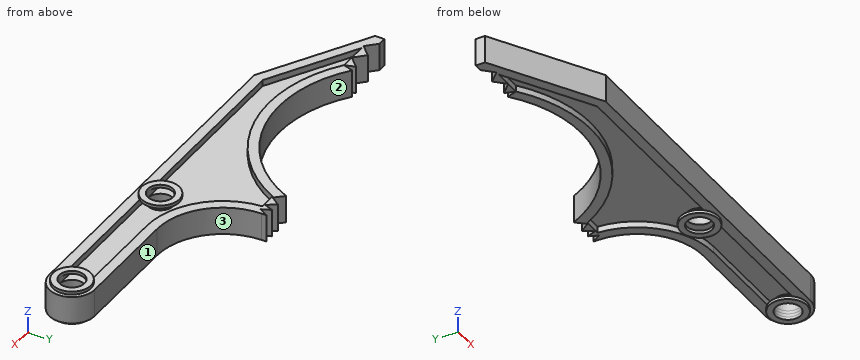
```python
from build123d import *

# Parameters (mm, degrees)
BOSS_EXTRUDE1_DEPTH     = 4
SKETCH3_R               = 2.5
CUT_EXTRUDE1_DEPTH      = 82.558227053
CUT_EXTRUDE2_DEPTH      = 1.25
SKETCH5_R               = 3.75
SKETCH5_R_2             = 2.5
BOSS_EXTRUDE2_DEPTH     = 0.625
CUT_EXTRUDE3_START      = -8
CUT_EXTRUDE3_DEPTH      = 8
CUT_EXTRUDE4_START      = -1.25
CUT_EXTRUDE4_DEPTH      = 1.25
CUT_EXTRUDE5_DEPTH      = 79.859241849
CUT_EXTRUDE5_DEPTH_BACK = 79.859241849
CUT_EXTRUDE6_DEPTH      = 79.859241849
CUT_EXTRUDE6_DEPTH_BACK = 79.859241849


# Read off the part's stored shape, not the designer's step: Cut-Extrude3
with BuildPart() as part:
    # Sketch1 → Boss-Extrude1 (new, symmetric)
    with BuildSketch(Plane.XY):
        with BuildLine():
            Line((0, 0), (70, 0))
            ThreePointArc((70, 0), (76.5, 6.5), (70, 13))
            Line((70, 13), (48.916352203, 13))
            ThreePointArc((48.916352203, 13), (41.053324797, 16.256972593), (37.796352203, 24.12))
            Line((37.796352203, 24.12), (37.796352203, 27.12))
            Line((37.796352203, 27.12), (27.786352203, 27.12))
            ThreePointArc((27.786352203, 27.12), (12.065558159, 13.089935965), (-8.483647797, 17.75))
            Line((-8.483647797, 17.75), (-22.083647797, 17.75))
            Line((-22.083647797, 17.75), (-22.083647797, 12.75))
            Line((-22.083647797, 12.75), (0, 0))
        make_face()
    extrude(amount=BOSS_EXTRUDE1_DEPTH, both=True)

    # Sketch3 → Cut-Extrude1 (cut, through all)
    with BuildSketch(Plane(origin=(0, 0, -4), x_dir=(-1, 0, 0), z_dir=(0, 0, -1))):
        with Locations((-70, 6.5)):
            Circle(SKETCH3_R)
        with Locations((-40, 6.5)):
            Circle(SKETCH3_R)
    extrude(amount=-CUT_EXTRUDE1_DEPTH, mode=Mode.SUBTRACT)

    # Sketch4 → Cut-Extrude2 (cut)
    with BuildSketch(Plane.XY.offset(4)):
        with BuildLine():
            Line((-20.083647797, 13.904700538), (0.535898385, 2))
            Line((0.535898385, 2), (70, 2))
            ThreePointArc((70, 2), (74.5, 6.5), (70, 11))
            Line((70, 11), (48.916352203, 11))
            ThreePointArc((48.916352203, 11), (39.639111234, 14.842759031), (35.796352203, 24.12))
            Line((35.796352203, 24.12), (35.796352203, 25.12))
            Line((35.796352203, 25.12), (29.119764251, 25.12))
            ThreePointArc((29.119764251, 25.12), (12.251390397, 11.074453376), (-9.195256898, 15.75))
            Line((-9.195256898, 15.75), (-20.083647797, 15.75))
            Line((-20.083647797, 15.75), (-20.083647797, 13.904700538))
        make_face()
    cut_extrude2 = extrude(amount=-CUT_EXTRUDE2_DEPTH, mode=Mode.SUBTRACT)

    # Sketch5 → Boss-Extrude2 (add, symmetric)
    # profile 1 of 2: a face of its own
    with BuildSketch(Plane.XY.offset(2.75)):
        with Locations((40, 6.5)):
            Circle(SKETCH5_R)
        with Locations(Location((40, 6.5, 0), (0, 0, 180))):
            Circle(SKETCH5_R_2, mode=Mode.SUBTRACT)
    # profile 2 of 2: a face of its own
    with BuildSketch(Plane.XY.offset(2.75)):
        with Locations((70, 6.5)):
            Circle(SKETCH5_R)
        with Locations(Location((70, 6.5, 0), (0, 0, 180))):
            Circle(SKETCH5_R_2, mode=Mode.SUBTRACT)
    boss_extrude2 = extrude(amount=BOSS_EXTRUDE2_DEPTH, both=True)

    # Mirror1: Cut-Extrude2, Boss-Extrude2 across plane
    add(cut_extrude2.mirror(Plane.XY), mode=Mode.SUBTRACT)
    add(boss_extrude2.mirror(Plane.XY))

    # Cut-Extrude3 outline → Cut-Extrude3 (cut)
    with BuildSketch(Plane.XY.offset(4).offset(CUT_EXTRUDE3_START)):
        with BuildLine():
            Line((-22.083647797, 12.75), (0, 0))
            Line((0, 0), (70, 0))
            ThreePointArc((70, 0), (76.5, 6.5), (70, 13))
            Line((70, 13), (48.916352203, 13))
            ThreePointArc((48.916352203, 13), (41.053324797, 16.256972594), (37.796352203, 24.12))
            Line((37.796352203, 24.12), (37.796352203, 27.12))
            Line((37.796352203, 27.12), (27.786352203, 27.12))
            ThreePointArc((27.786352203, 27.12), (12.065558159, 13.089935965), (-8.483647797, 17.75))
            Line((-8.483647797, 17.75), (-22.083647797, 17.75))
            Line((-22.083647797, 17.75), (-22.083647797, 12.75))
        make_face()
        with BuildLine():
            Line((0.535898385, 2), (-20.083647797, 13.904700538))
            Line((-20.083647797, 13.904700538), (-20.083647797, 15.75))
            Line((-20.083647797, 15.75), (-9.195256898, 15.75))
            ThreePointArc((-9.195256898, 15.75), (12.251390397, 11.074453376), (29.119764251, 25.12))
            Line((29.119764251, 25.12), (35.796352203, 25.12))
            Line((35.796352203, 25.12), (35.796352203, 24.12))
            ThreePointArc((35.796352203, 24.12), (39.639111234, 14.842759031), (48.916352203, 11))
            Line((48.916352203, 11), (70, 11))
            ThreePointArc((70, 11), (74.5, 6.5), (70, 2))
            Line((70, 2), (0.535898385, 2))
        make_face(mode=Mode.SUBTRACT)
    cut_extrude3 = extrude(amount=CUT_EXTRUDE3_DEPTH, mode=Mode.SUBTRACT)

    # Sketch8 → Cut-Extrude4 (cut)
    with BuildSketch(Plane.XY.offset(2.75).offset(CUT_EXTRUDE4_START)):
        with BuildLine():
            Line((-15.815698604, 13.75), (1.07179677, 4))
            Line((1.07179677, 4), (70, 4))
            ThreePointArc((70, 4), (72.5, 6.5), (70, 9))
            Line((70, 9), (48.916352203, 9))
            ThreePointArc((48.916352203, 9), (38.584498546, 13.080652193), (33.829457228, 23.12))
            Line((33.829457228, 23.12), (30.37941216, 23.12))
            ThreePointArc((30.37941216, 23.12), (12.433656393, 9.061817656), (-9.875614934, 13.75))
            Line((-9.875614934, 13.75), (-15.815698604, 13.75))
        make_face()
    cut_extrude4 = extrude(amount=CUT_EXTRUDE4_DEPTH, mode=Mode.SUBTRACT)

    # Mirror2: Cut-Extrude3, Cut-Extrude4 across plane
    add(cut_extrude3.mirror(Plane.XY), mode=Mode.SUBTRACT)
    add(cut_extrude4.mirror(Plane.XY), mode=Mode.SUBTRACT)

    # Sketch9 → Cut-Extrude5 (cut, two sides: drawn at the far end of the back side and taken through both)
    with BuildSketch(Plane.XY.offset(2.75).offset(-CUT_EXTRUDE5_DEPTH_BACK)):
        Polygon((-158.483427763, 155.749779966), (-18.483647797, 15.75), (-16.482535606, 13.748887809), (-14.481423415, 15.75), (-12.480311224, 13.748887809), (-10.479199033, 15.75), (-9.839204987, 13.748887809), (-9.195256898, 15.75), (51.453981857, 204.221606933), (-37.628855278, 590.05026742), (-247.566264898, 541.578440454), align=None)
    extrude(amount=CUT_EXTRUDE5_DEPTH + CUT_EXTRUDE5_DEPTH_BACK, mode=Mode.SUBTRACT)

    # Sketch11 → Cut-Extrude6 (cut, two sides: drawn at the far end of the back side and taken through both)
    with BuildSketch(Plane.XY.offset(2.75).offset(-CUT_EXTRUDE6_DEPTH_BACK)):
        Polygon((-58.744613453, 122.187820827), (29.099875124, 25.075811319), (30.688127166, 23.32), (32.002745662, 25.12), (33.242951791, 23.32), (33.9290832, 25.12), (34.735542366, 23.32), (35.796352203, 25.12), (102.282124161, 137.934177705), (76.793604285, 398.587053406), (-84.233133328, 382.840696528), align=None)
    extrude(amount=CUT_EXTRUDE6_DEPTH + CUT_EXTRUDE6_DEPTH_BACK, mode=Mode.SUBTRACT)


solid = part.part
```
Here's how the part is built. I have some questions about the finished solid (model axes, mm). Face numbers are marked on the shaded views. Give positions to 0.01 mm unless a question says otherwise; leave off trailing zeros. Loops run counter-clockwise (first coordinate to the right, second up) from the corner with the lowest first, then second, coordinate; pieces in that order, holes last. Notation, with made-up numbers: M -17,-9.75 L -6,-9.75 A25 ccw -6,2.25 Z; hole C 62,23 d5. An arc over 180 degrees is marked long. Put each result on its own line as item: value. Start each with the question number.
(1) I want a section at A-A on x = 50. Please give me the cut outline in (y, z).
(2) If we mould it in two halves opening along X, with no side actions, what happens to the marked faces 1, 2 and 3? For each: +X half, -X half, draft (parallel to the pull), parting line (faces both ways), or undercut.
(3) I want a section at B-B on y = 18.5. Please give me the cut outline in (x, z), then the cut area to 3 significant figures.
(4) Will these pins go through, and if not, where does the flat tip stop? pin 1 Ø4 at (x, z) = (-4, -1) entering from -Y; pin 2 Ø5.5 at (x, y) = (17.5, 15.5) entering from -Z; pin 3 Ø3 at (y, z) = (10, -1) entering from +X.
(5) I need wall thicknesses on line 1 along X through (y, z) = (6.5, -3.1); line 2 along Y through (x, z) = (40, -3.1); line 3 along X through (y, z) = (6.5, 0.85). Which ranges of each line are inside material? Lowest first, please. Write a range as [from, to].
(6) I want a section at C-C on y = 6.5. State how many separate pieces and enclosed holes the cut face has, then the cut area to 3 significant figures.
Answer block:
1. outline: M 2,-2.75 L 4,-2.75 L 4,-1.5 L 9,-1.5 L 9,-2.75 L 11,-2.75 L 11,2.75 L 9,2.75 L 9,1.5 L 4,1.5 L 4,2.75 L 2,2.75 Z
2. face 1: draft
2. face 2: undercut
2. face 3: +X half
3. outline: M 24.77,-2.75 L 27.4,-2.75 L 27.4,-1.5 L 34.88,-1.5 L 34.88,-2.75 L 37.06,-2.75 L 37.06,2.75 L 34.88,2.75 L 34.88,1.5 L 27.4,1.5 L 27.4,2.75 L 24.77,2.75 Z
3. area: 48.9 mm^2
4. pin 1: y = 3.46
4. pin 2: z = -2.75
4. pin 3: x = 74.03
5. line 1: [36.25, 37.5], [42.5, 43.75], [66.25, 67.5], [72.5, 73.75]
5. line 2: [2.75, 4], [9, 10.25]
5. line 3: [-7.26, 37.5], [42.5, 67.5], [72.5, 74.5]
6. separate pieces: 9
6. enclosed holes: 0
6. area: 237 mm^2
